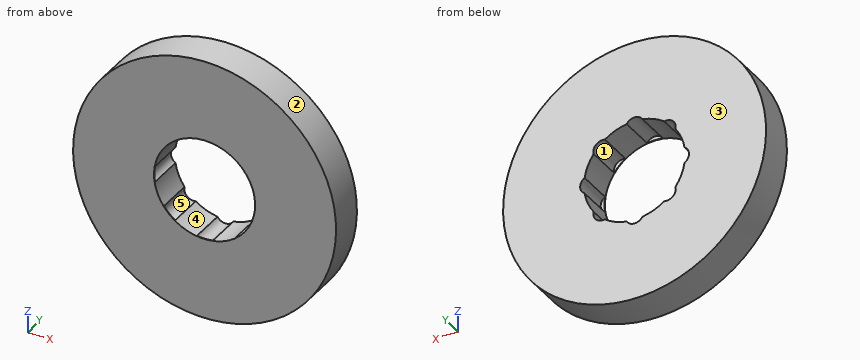
```python
from build123d import *

# Parameters (mm, degrees)
SKETCH1_R           = 32.5
BOSS_EXTRUDE1_DEPTH = 9
SKETCH2_R           = 12.5
CUT_EXTRUDE1_DEPTH  = 47.834816109
SKETCH3_R           = 2.293323558
CUT_EXTRUDE2_DEPTH  = 8.845206
CIRPATTERN1_START   = 0.154793712
CIRPATTERN1_DEPTH   = 8.845206288


# Read off the part's stored shape, not the designer's step: CirPattern1
with BuildPart() as part:
    # Sketch1 → Boss-Extrude1 (new body)
    with BuildSketch(Plane(origin=(0, 0, 0), x_dir=(1, 0, 0), z_dir=(0, 1, 0))):
        with Locations(Location((0, 0, 0), (0, 0, 270))):
            Circle(SKETCH1_R)
    extrude(amount=BOSS_EXTRUDE1_DEPTH)

    # Sketch2 → Cut-Extrude1 (cut, through all)
    with BuildSketch(Plane(origin=(0, 0, 0), x_dir=(1, 0, 0), z_dir=(0, 1, 0))):
        with Locations(Location((0, 0, 0), (0, 0, 270))):
            Circle(SKETCH2_R)
    extrude(amount=CUT_EXTRUDE1_DEPTH, mode=Mode.SUBTRACT)

    # Sketch3 → Cut-Extrude2 (cut)
    with BuildSketch(Plane(origin=(0, 9, 0), x_dir=(1, 0, 0), z_dir=(0, 1, 0))):
        with Locations((-11.154965368, 0)):
            Circle(SKETCH3_R)
    extrude(amount=-CUT_EXTRUDE2_DEPTH, mode=Mode.SUBTRACT)

    # CirPattern1 outline → CirPattern1 (cut)
    with BuildSketch(Plane(origin=(0, 0, 0), x_dir=(1, 0, 0), z_dir=(0, 1, 0)).offset(CIRPATTERN1_START)):
        with BuildLine():
            ThreePointArc((-7.343422829, -10.115539588), (-8.838834765, -8.838834765), (-10.115539588, -7.343422829))
            ThreePointArc((-10.115539588, -7.343422829), (-9.509376295, -9.509376295), (-7.343422829, -10.115539588))
        make_face()
        with BuildLine():
            ThreePointArc((-7.343422829, 10.115539588), (-9.509376295, 9.509376295), (-10.115539588, 7.343422829))
            ThreePointArc((-10.115539588, 7.343422829), (-8.838834765, 8.838834765), (-7.343422829, 10.115539588))
        make_face()
        with BuildLine():
            ThreePointArc((1.960182558, -12.345350718), (0, -12.5), (-1.960182558, -12.345350718))
            ThreePointArc((-1.960182558, -12.345350718), (0, -13.448288926), (1.960182558, -12.345350718))
        make_face()
        with BuildLine():
            ThreePointArc((1.960182558, 12.345350718), (0, 13.448288926), (-1.960182558, 12.345350718))
            ThreePointArc((-1.960182558, 12.345350718), (0, 12.5), (1.960182558, 12.345350718))
        make_face()
        with BuildLine():
            ThreePointArc((10.115539588, -7.343422829), (8.838834765, -8.838834765), (7.343422829, -10.115539588))
            ThreePointArc((7.343422829, -10.115539588), (9.509376295, -9.509376295), (10.115539588, -7.343422829))
        make_face()
        with BuildLine():
            ThreePointArc((10.115539588, 7.343422829), (9.509376295, 9.509376295), (7.343422829, 10.115539588))
            ThreePointArc((7.343422829, 10.115539588), (8.838834765, 8.838834765), (10.115539588, 7.343422829))
        make_face()
        with BuildLine():
            ThreePointArc((12.345350718, 1.960182558), (12.5, 0), (12.345350718, -1.960182558))
            ThreePointArc((12.345350718, -1.960182558), (13.448288926, 0), (12.345350718, 1.960182558))
        make_face()
    extrude(amount=CIRPATTERN1_DEPTH, mode=Mode.SUBTRACT)


solid = part.part
```
CAD build for the part. Positions are in the model's coordinates, mm. Face numbers are marked on the shaded views. A direction names the side the tool comes from. Give positions to 0.01 mm unless a question says otherwise; leave off trailing zeros. Loops run counter-clockwise (first coordinate to the right, second up) from the corner with the lowest first, then second, coordinate; pieces in that order, holes last. Notation, with made-up numbers: (-6.5, 88.5) - (23.5, 88.5) arc R25 ccw to (23.5, 102.5) - close; hole circle Ø8 at (83.25, -24). An arc over 180 degrees is marked (long way). Put each result on its own line as item: value.
Q1. Slice it at B-B (x = 0). Give the cut face in (y, z).
Filled in:
outline: (0, -32.5) - (9, -32.5) - (9, -13.45) - (0.15, -13.45) - (0.15, -12.5) - (0, -12.5) - close; (0, 12.5) - (0.15, 12.5) - (0.15, 13.45) - (9, 13.45) - (9, 32.5) - (0, 32.5) - close
Q2. Slice it at C-C (y = 7). Give the cut face in (x, z), plus the area to 3 significant figures.
Filled in:
outline: circle Ø65 at (0, 0); hole (-12.35, -1.96) arc R12.5 ccw to (-10.12, -7.34) arc R2.29 ccw to (-7.34, -10.12) arc R12.5 ccw to (-1.96, -12.35) arc R2.29 ccw to (1.96, -12.35) arc R12.5 ccw to (7.34, -10.12) arc R2.29 ccw to (10.12, -7.34) arc R12.5 ccw to (12.35, -1.96) arc R2.29 ccw to (12.35, 1.96) arc R12.5 ccw to (10.12, 7.34) arc R2.29 ccw to (7.34, 10.12) arc R12.5 ccw to (1.96, 12.35) arc R2.29 ccw to (-1.96, 12.35) arc R12.5 ccw to (-7.34, 10.12) arc R2.29 ccw to (-10.12, 7.34) arc R12.5 ccw to (-12.35, 1.96) arc R2.29 ccw to start
area: 2,810 mm²
Q3. Slice it at D-D (z = 19). Give the cut face in (x, y), plus the area to 3 significant figures.
Filled in:
outline: (-26.37, 0) - (26.37, 0) - (26.37, 9) - (-26.37, 9) - close
area: 475 mm²
Q4. Flat gauge pins, fed straight in: pin 1 (4 mm diameter, centred on y = 1.5, z = 14, fed in from +X); pin 2 (3 mm diameter, centred on x = 12, y = 3, fed in from -Z); pin 3 (2 mm diameter, centred on y = 2.5, z = 22, fed in from +X). Where does each tip first touch, or does it go through?
Filled in:
pin 1: stops at x = 30.2
pin 2: stops at z = -30.76
pin 3: stops at x = 24.8
Q5. Slice it at A-A (z = 0). Give the cut face in (x, y).
Filled in:
outline: (-32.5, 0) - (-12.5, 0) - (-12.5, 0.15) - (-13.45, 0.15) - (-13.45, 9) - (-32.5, 9) - close; (12.5, 0) - (32.5, 0) - (32.5, 9) - (13.45, 9) - (13.45, 0.15) - (12.5, 0.15) - close
Q6. Mould opens along X. For the marked faces 1, 2 and 3 say: pulls with the +X half, pulls with the -X half, needs draft (parallel to the pull), parting line crosses it, or undercut.
Filled in:
face 1: undercut
face 2: parting line crosses it
face 3: needs draft
Q7. Probe line 1 along X through (y, z) = (6.75, 0); line 2 along X through (y, z) = (2.25, -7); line 3 along Z through (x, y) = (6.5, 2.5). List the from-to ranges inside material, lowest first.
Filled in:
line 1: x = -32.5 to -13.45, 13.45 to 32.5
line 2: x = -31.74 to -10.36, 10.36 to 31.74
line 3: z = -31.84 to -10.68, 10.68 to 31.84
Q8. Tool access for the marked faces 4 and 5: list every direction of +Z, -Z, +X, -X, +Y, -Y with a clear straight run to the whole face (end or side of a thin tool).
Filled in:
face 4: +Y, -Y
face 5: +Y
